Input: dimensioned drawing with shaded views. Units: mm. Origin: part minimum x, y, z. Coordinates: 2 decimals unless noted, no trailing zeros. Write each loop counter-clockwise with the first axis right and the second up, starting at its lowest first coordinate (ties: lowest second). Pieces come first, ordered by that corner, then holes. Notation, with made-up numbers: (72.25, 38) - (127.25, 38) arc R15 cw to (127.25, 67) - close; hole circle Ø2 at (36, 8.25). An arc over 180 degrees is marked (long way). One line per question, with ' | ' between items.
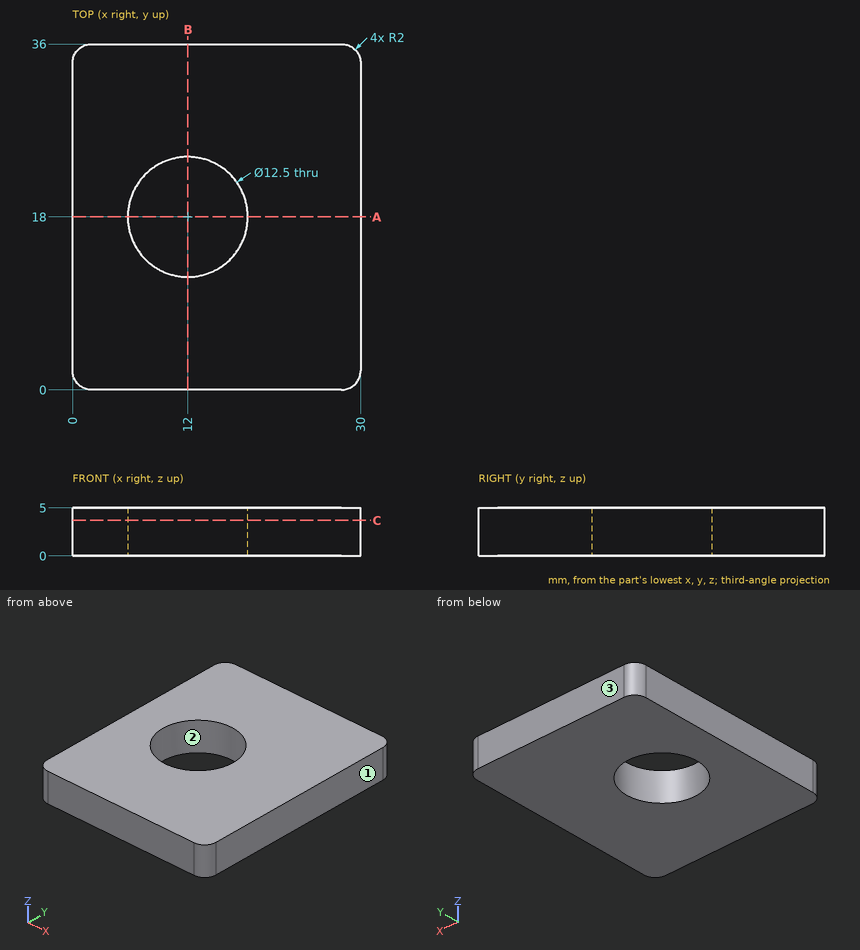
Item 1: Cut plane B-B on x = 12. Return loops of the section in (y, z), and give its area (4 significant figures).
Check sheet entries:
outline: (0, 0) - (11.75, 0) - (11.75, 5) - (0, 5) - close; (24.25, 0) - (36, 0) - (36, 5) - (24.25, 5) - close | area: 117.5 mm²
Item 2: Cut plane C-C on z = 3.7. Return loops of the section in (x, y), and give its area (3 significant figures).
Check sheet entries:
outline: (0, 2) arc R2 ccw to (2, 0) - (28, 0) arc R2 ccw to (30, 2) - (30, 34) arc R2 ccw to (28, 36) - (2, 36) arc R2 ccw to (0, 34) - close; hole circle Ø12.5 at (12, 18) | area: 954 mm²
Item 3: Ray query, line 1 along Y through (x, z) = (12, 1.7); line 2 along X through (y, z) = (15, 0.3); line 3 along X through (y, z) = (14, 2.25). Return the intervals inside material, ascending. Write a range as [from, to].
Check sheet entries:
line 1: [0, 11.75], [24.25, 36] | line 2: [0, 6.52], [17.48, 30] | line 3: [0, 7.2], [16.8, 30]
Item 4: Cut plane A-A on y = 18. Return loops of the section in (x, z).
Check sheet entries:
outline: (0, 0) - (5.75, 0) - (5.75, 5) - (0, 5) - close; (18.25, 0) - (30, 0) - (30, 5) - (18.25, 5) - close
Item 5: Mould query, pull axis X, two halves, no side actions, for the marked faces 1, 2 and 3. Classes: pulls with the +X half, pulls with the -X half, needs draft (parallel to the pull), parting line crosses it, or undercut.
Check sheet entries:
face 1: pulls with the +X half | face 2: undercut | face 3: needs draft
